from build123d import *

# Parameters (mm, degrees)
BOSS_EXTRUDE1_DEPTH = 44.45
SKETCH2_R           = 13.97
CUT_EXTRUDE1_DEPTH  = 33.02
SKETCH4_R           = 1.524
CUT_EXTRUDE2_DEPTH  = 11.43
CUT_EXTRUDE4_DEPTH  = 44.45
SKETCH6_W           = 44.799560936
SKETCH6_H           = 27.686
CUT_EXTRUDE5_DEPTH  = 22.225


with BuildPart() as part:
    # Sketch1 → Boss-Extrude1 (new body)
    with BuildSketch(Plane(origin=(0, 0, 0), x_dir=(1, 0, 0), z_dir=(0, 1, 0))):
        with BuildLine():
            Line((-5.43632278, -18.484519804), (50.753878982, -98.550855941))
            ThreePointArc((50.753878982, -98.550855941), (67.749452613, -101.528977989), (70.727574662, -84.533404358))
            Line((70.727574662, -84.533404358), (19.143911472, -2.177551677))
            ThreePointArc((19.143911472, -2.177551677), (18.167371728, -0.148266421), (17.661854227, 2.046290613))
            ThreePointArc((17.661854227, 2.046290613), (-9.829221355, 14.816032112), (-8.751716681, -15.476945924))
            ThreePointArc((-8.751716681, -15.476945924), (-6.926324763, -16.795874604), (-5.43632278, -18.484519804))
        make_face()
    extrude(amount=BOSS_EXTRUDE1_DEPTH)

    # Sketch2 → Cut-Extrude1 (cut)
    with BuildSketch(Plane(origin=(0, 44.45, 0), x_dir=(1, 0, 0), z_dir=(0, 1, 0))):
        Circle(SKETCH2_R)
    extrude(amount=-CUT_EXTRUDE1_DEPTH, mode=Mode.SUBTRACT)

    # Sketch4 → Cut-Extrude2 (cut)
    with BuildSketch(Plane.XZ):
        Circle(SKETCH4_R)
    extrude(amount=-CUT_EXTRUDE2_DEPTH, mode=Mode.SUBTRACT)

    # Sketch5 → Cut-Extrude4 (cut)
    with BuildSketch(Plane(origin=(0, 44.45, 0), x_dir=(1, 0, 0), z_dir=(0, 1, 0))):
        with BuildLine():
            Line((-2.419955599, -13.758804995), (53.761320997, -93.799464422))
            ThreePointArc((53.761320997, -93.799464422), (57.042861973, -95.884776857), (60.837800413, -95.038915544))
            Line((60.837800413, -95.038915544), (64.500597561, -92.467964465))
            ThreePointArc((64.500597561, -92.467964465), (66.561253196, -89.317108071), (65.887093565, -85.613095861))
            Line((65.887093565, -85.613095861), (13.761291875, -2.405773456))
            ThreePointArc((13.761291875, -2.405773456), (8.023671754, -11.435977946), (-2.419955599, -13.758804995))
        make_face()
    extrude(amount=-CUT_EXTRUDE4_DEPTH, mode=Mode.SUBTRACT)

    # Sketch6 → Cut-Extrude5 (cut, symmetric)
    with BuildSketch(Plane(origin=(63.31167299, 0, 90.199232956), x_dir=(-0.8184971, 0, 0.574510659), z_dir=(-0.574510659, 0, -0.8184971))):
        with Locations((1.370623881, 22.225)):
            Rectangle(SKETCH6_W, SKETCH6_H)
    extrude(amount=CUT_EXTRUDE5_DEPTH, both=True, mode=Mode.SUBTRACT)


solid = part.part
For this review, take the finished solid that the model builds, in its own axes (mm). A direction names the side the tool comes from. Give positions to 0.01 mm unless a question says otherwise; leave off trailing zeros. Loops run counter-clockwise (first coordinate to the right, second up) from the corner with the lowest first, then second, coordinate; pieces in that order, holes last. Notation, with made-up numbers: M -2.75,55.25 L 45.25,55.25 A29 cw 45.25,88.25 Z; hole C 77,-4.5 d3. An arc over 180 degrees is marked long. Put each result on its own line as item: value. Start each with the question number.
(1) Add section A-A, the plane y = 40.5. Write out the cut boundary in (x, z).
(2) Add section D-D, the plane x = 39.5. Write out the cut boundary in (y, z).
(3) For pin 1 (3 mm diameter, centred on y = 24.5, z = 48.5, fed in from -X); pin 2 (1.5 mm diameter, centred on y = 10.5, z = 46.5, fed in from -X); pin 3 (2.5 mm diameter, centred on x = 0, z = 0, fed in from -Y); pin 4 (14 mm diameter, centred on x = 4, z = 6, fed in from +Y), all flat-tipped, find the tip position at first contact; note any pin that passes through.
(4) Add section C-C, the plane y = 5. Write out the cut boundary in (x, z), then the cut area to 3 significant figures.
(5) The part is to be moulded in two halves that separate along Y. For faces 5 (the flat face through (20.6, 44.45, 47.2)), 6 (the flat face through (58.1, 8.382, 96.4)), 7 (the cylindrical face through (67.5, 4.1, 101.7)), say which applies: +Y half, -Y half, draft (parallel to the pull), parting line (faces both ways), or undercut.
(6) Machinability: for faces 1 (the cylindrical face through (56.988, 40.318, 95.875)), 2 (the cylindrical face through (-7.642, 28.171, -11.694)), 3 (the cylindrical face through (18.18, 21.91, 0.18)), 4 (the flat face through (57.22, 22.42, 67.32)), which of the approach directions +Z, -Z, +X, -X, +Y, -Y give a long, thin tool a straight path to every point of the face, cutting with its end or side? Answer none if there is none.
(7) Wall thickness on L1, parallel to Z at x = 0, y = 7.5; L2, parallel to Z at x = 0, y = 20.5; L3, parallel to X at y = 33, z = 0: over which ranges is each line inside the solid? List them lowest first.
(8) Add section B-B, the plane z = 35.5. Write out the cut boundary in (x, y), then the cut area to 3 significant figures.
Result:
1. outline: M -8.75,15.48 A17.78 ccw long 17.66,-2.05 A10.16 cw 19.14,2.18 L 70.73,84.53 A12.2 ccw 50.75,98.55 L -5.44,18.48 A10.16 cw Z; hole M -2.42,13.76 A13.97 ccw long 13.76,2.41 L 65.89,85.61 A5.08 ccw 64.5,92.47 L 60.84,95.04 A5.08 ccw 53.76,93.8 Z
2. outline: M 0,34.68 L 44.45,34.68 L 44.45,43.49 L 0,43.49 Z; M 0,73.48 L 44.45,73.48 L 44.45,82.52 L 36.07,82.52 L 36.07,79.76 L 8.38,79.76 L 8.38,82.52 L 0,82.52 Z
3. pin 1: stops at x = 14.58
3. pin 2: stops at x = 13.7
3. pin 3: passes through
3. pin 4: stops at y = 11.43
4. outline: M -8.75,15.48 A17.78 ccw long 17.66,-2.05 A10.16 cw 19.14,2.18 L 70.73,84.53 A12.2 ccw 50.75,98.55 L -5.44,18.48 A10.16 cw Z; hole M -2.42,13.76 A13.97 cw 13.76,2.41 L 65.89,85.61 A5.08 ccw 64.5,92.47 L 60.84,95.04 A5.08 ccw 53.76,93.8 Z; hole C 0,0 d3.05
4. area: 2,070 mm^2
5. face 5: +Y half
5. face 6: undercut
5. face 7: draft
6. face 1: +Y, -Y
6. face 2: +Y
6. face 3: -Z, +X, +Y, -Y
6. face 4: +Z, +X
7. L1: z = -17.78 to -1.52, 1.52 to 13.97, 17.21 to 26.23
7. L2: z = -17.78 to -13.97, 17.21 to 26.23
7. L3: x = -17.78 to -13.97, 13.97 to 18.12
8. outline: M 6.51,0 L 12.84,0 L 12.84,44.45 L 6.51,44.45 Z; M 34.49,0 L 40.02,0 L 40.02,44.45 L 34.49,44.45 Z
8. area: 527 mm^2
